Part model, mm, in its own coordinate system. A direction names the side the tool comes from. Give positions to 0.01 mm unless a question says otherwise; leave off trailing zeros. Write each loop counter-clockwise with the first axis right and the second up, starting at its lowest first coordinate (ties: lowest second). Pieces come first, ordered by that corner, then holes. Notation, with made-up numbers: M 49.25,-14 L 95.25,-14 A10 cw 95.25,-3 Z; hole C -8,-12 d4. An arc over 180 degrees is marked long. Write item = value, one per line. Start each with the question number.
from build123d import *

# Parameters (mm, degrees)
SKETCH2_W           = 25
SKETCH2_H           = 18
BOSS_EXTRUDE1_DEPTH = 1.5
BOSS_EXTRUDE2_DEPTH = 5
SKETCH5_R           = 1
CUT_EXTRUDE1_DEPTH  = 1.5


with BuildPart() as part:
    # Sketch2 → Boss-Extrude1 (new body)
    with BuildSketch(Plane(origin=(0, 0, 0), x_dir=(1, 0, 0), z_dir=(0, 1, 0))):
        with Locations((12.5, 9)):
            Rectangle(SKETCH2_W, SKETCH2_H)
    extrude(amount=BOSS_EXTRUDE1_DEPTH)

    # Sketch3 → Boss-Extrude2 (add)
    with BuildSketch(Plane(origin=(0, 1.5, 0), x_dir=(1, 0, 0), z_dir=(0, 1, 0))):
        Polygon((3.438353886, 3.85), (9.385061659, 3.85), (11.25, 7.08016796), (11.25, 10.91983204), (9.385061659, 14.15), (3.438353886, 14.15), (0.465, 9), align=None)
        Polygon((13.75, 11.156403255), (13.75, 6.843596745), (15.478353886, 3.85), (21.425061659, 3.85), (24.398415545, 9), (21.425061659, 14.15), (15.478353886, 14.15), align=None)
    extrude(amount=BOSS_EXTRUDE2_DEPTH)

    # Sketch5 → Cut-Extrude1 (cut)
    with BuildSketch(Plane.XZ):
        with Locations((4.5, -2.25)):
            Circle(SKETCH5_R)
        with Locations((19.5, -2.25)):
            Circle(SKETCH5_R)
    extrude(amount=-CUT_EXTRUDE1_DEPTH, mode=Mode.SUBTRACT)


solid = part.part
Q1. Two-plate mould, pull along X, no slides. Class faces 5 (the face through (1.97, 3.96, -11.61)), 6 (the face through (14.626, 3.965, -12.674)), 7 (the face through (22.93, 3.96, -11.54)): +X half, -X half, draft (parallel to the pull), parting line (faces both ways), or undercut.
Q2. Tool access for faces 1 (the face through (18, 4, -3.85)), 2 (the face through (10.304, 3.965, -5.442)), 3 (the face through (1.93, 3.96, -6.46)), 4 (the face through (22.89, 3.96, -6.39)): list every direction of +Z, -Z, +X, -X, +Y, -Y with a clear straight run to the whole face (end or side of a thin tool).
Q3. Slice it at B-B (y = 3.25). Give the cut face in (x, z) (3 decimals), and give its area (3 significant figures).
Q4. Slice it at C-C (x = 17.5). Give the cut face in (y, z).
Q5. Slice it at D-D (z = -7.75). Give the cut face in (x, y), and give its area (3 significant figures).
Q6. Probe line 1 along Z through (x, y) = (4.5, 0.4); line 2 along Y through (x, z) = (3.25, -16.5); line 3 along Z through (x, y) = (15.5, 2). List the from-to ranges inside material, lowest first.
Q7. Slice it at A-A (x = 4.5). Give the cut face in (y, z).
Q8. Drop flat-ended pins along their axis: P1, Ø3.5, axis at y = 4.5, z = -10, coming from the -X side (3 decimals); P2, Ø1.5, axis at x = 18.5, y = 4.5, coming from the -Z side; P3, Ø1.5, axis at y = 4.5, z = -9, coming from the +X side. Give the stop position or say it passes through.
Working result:
q1.face_5 = -X half
q1.face_6 = undercut
q1.face_7 = +X half
q2.face_1 = +Z, +X, -X, +Y
q2.face_2 = +Z, +Y
q2.face_3 = +Z, -X, +Y
q2.face_4 = +Z, +X, +Y
q3.outline = M 0.465,-9 L 3.438,-14.15 L 9.385,-14.15 L 11.25,-10.92 L 11.25,-7.08 L 9.385,-3.85 L 3.438,-3.85 Z; M 13.75,-11.156 L 15.478,-14.15 L 21.425,-14.15 L 24.398,-9 L 21.425,-3.85 L 15.478,-3.85 L 13.75,-6.844 Z
q3.area = 179 mm2
q4.outline = M 0,-18 L 1.5,-18 L 1.5,-14.15 L 6.5,-14.15 L 6.5,-3.85 L 1.5,-3.85 L 1.5,0 L 0,0 Z
q5.outline = M 0,0 L 25,0 L 25,1.5 L 23.68,1.5 L 23.68,6.5 L 13.75,6.5 L 13.75,1.5 L 11.25,1.5 L 11.25,6.5 L 1.19,6.5 L 1.19,1.5 L 0,1.5 Z
q5.area = 137 mm2
q6.line_1 = -18 to -3.25, -1.25 to 0
q6.line_2 = 0 to 1.5
q6.line_3 = -14.15 to -3.85
q7.outline = M 0,-18 L 1.5,-18 L 1.5,-14.15 L 6.5,-14.15 L 6.5,-3.85 L 1.5,-3.85 L 1.5,-3.25 L 0,-3.25 Z; M 0,-1.25 L 1.5,-1.25 L 1.5,0 L 0,0 Z
q8.P1 = 0.465
q8.P2 = -14.15
q8.P3 = 24.4
